from build123d import *

# Parameters (mm, degrees)
ESQUISSE1_R             = 20
ESQUISSE1_R_2           = 8.5
BOSS_EXTRU_1_DEPTH      = 13.25
ESQUISSE2_R             = 17
ENL_V_MAT_EXTRU_1_DEPTH = 1
ESQUISSE3_OUTSIDE_W     = 53.62
ESQUISSE3_OUTSIDE_H     = 53.62
ESQUISSE3_OUTSIDE_R     = 16
ENL_V_MAT_EXTRU_2_DEPTH = 1


with BuildPart() as part:
    # Esquisse1 → Boss.-Extru.1 (new body)
    with BuildSketch(Plane.XY):
        Circle(ESQUISSE1_R)
        Circle(ESQUISSE1_R_2, mode=Mode.SUBTRACT)
    extrude(amount=BOSS_EXTRU_1_DEPTH)

    # Esquisse2 → Enlèv. mat.-Extru.1 (cut)
    with BuildSketch(Plane(origin=(0, 0, 0), x_dir=(-1, 0, 0), z_dir=(0, 0, -1))):
        Circle(ESQUISSE2_R)
    extrude(amount=-ENL_V_MAT_EXTRU_1_DEPTH, mode=Mode.SUBTRACT)

    # Esquisse3 outside → Enlèv. mat.-Extru.2 (cut)
    with BuildSketch(Plane.XY.offset(13.25)):
        Rectangle(ESQUISSE3_OUTSIDE_W, ESQUISSE3_OUTSIDE_H)
        Circle(ESQUISSE3_OUTSIDE_R, mode=Mode.SUBTRACT)
    extrude(amount=-ENL_V_MAT_EXTRU_2_DEPTH, mode=Mode.SUBTRACT)


solid = part.part
Geometry check sheet. Reference: the model listing, model coordinates, mm. A direction names the side the tool comes from. Round coordinates to 2 decimals unless told otherwise and drop trailing zeros. Loops run counter-clockwise (first coordinate to the right, second up) from the corner with the lowest first, then second, coordinate; pieces in that order, holes last. Notation, with made-up numbers: (-13, 40.5) -> (15, 40.5) arc R23 ccw to (15, 78.5) -> close; hole circle Ø1 at (-29.5, 47). An arc over 180 degrees is marked (long way). Answer as a JSON object with one key per item and string values. Group by question number.
Item 1: Thickness scan on line 1 along Y through (x, z) = (0, 0.6); line 2 along Y through (x, z) = (0, 8). Record the ranges inside material, lowest first.
Item 2: Cross-section at D-D, the plane y = 9. Record the cut outline in (x, z), plus the area to 3 significant figures.
Item 3: Set-up check for faces 4 (the face through (-3.47, -15.62, 12.76)), 5 (the face through (-9.139, 14.334, 0.493)), 6 (the face through (4.57, 7.167, 7.039)): record each of +Z, -Z, +X, -X, +Y, -Y from which the full face is reachable in a straight line by a thin tool's end or side.
Item 4: Release check for a two-part mould opening along X. For faces 1 (the face through (-4.336, -19.524, 6.039)), 2 (the face through (7, -7, 13.25)), 3 (the face through (8, -4, 1)) record: pulls with the +X half, pulls with the -X half, needs draft (parallel to the pull), parting line crosses it, or undercut.
Item 5: Cross-section at C-C, the plane z = 5.5. Record the cut outline in (x, y), plus the area to 3 significant figures.
Item 6: Cross-section at A-A, the plane y = 0. Record the cut outline in (x, z), plus the area to 3 significant figures.
Item 7: Depth check by flat-ended pin: pin 1 Ø2 at (y, z) = (14.5, 9) entering from -X; pin 2 Ø6 at (x, z) = (-10, 3.5) entering from -Y (3 decimals); pin 3 Ø2 at (x, y) = (0.5, -15.5) entering from -Z. Enter the tip coordinate at first touch or a pass-through.
Determined:
{
 "1": {"line 1": "y = -20 to -17, 17 to 20", "line 2": "y = -20 to -8.5, 8.5 to 20"},
 "2": {"outline": "(-17.86, 0) -> (-14.42, 0) -> (-14.42, 1) -> (14.42, 1) -> (14.42, 0) -> (17.86, 0) -> (17.86, 12.25) -> (13.23, 12.25) -> (13.23, 13.25) -> (-13.23, 13.25) -> (-13.23, 12.25) -> (-17.86, 12.25) -> close", "area": "435 mm²"},
 "3": {"face 4": "+Z", "face 5": "-Z", "face 6": "+Z, -Z"},
 "4": {"face 1": "parting line crosses it", "face 2": "needs draft", "face 3": "undercut"},
 "5": {"outline": "circle Ø40 at (0, 0); hole circle Ø17 at (0, 0)", "area": "1,030 mm²"},
 "6": {"outline": "(-20, 0) -> (-17, 0) -> (-17, 1) -> (-8.5, 1) -> (-8.5, 13.25) -> (-16, 13.25) -> (-16, 12.25) -> (-20, 12.25) -> close; (8.5, 1) -> (17, 1) -> (17, 0) -> (20, 0) -> (20, 12.25) -> (16, 12.25) -> (16, 13.25) -> (8.5, 13.25) -> close", "area": "280 mm²"},
 "7": {"pin 1": "stops at x = -14.76", "pin 2": "stops at y = -18.735", "pin 3": "stops at z = 1"}
}
